Build history of the part. All positions in model axes, mm. Round coordinates to 2 decimals unless told otherwise and drop trailing zeros. Loops run counter-clockwise (first coordinate to the right, second up) from the corner with the lowest first, then second, coordinate; pieces in that order, holes last. Notation, with made-up numbers: (78, 64) - (114, 64) arc R11 ccw to (114, 80) - close; hole circle Ø7 at (63.25, -1). An arc over 180 degrees is marked (long way). Put each result on its own line as item: value. Start each with the question number.
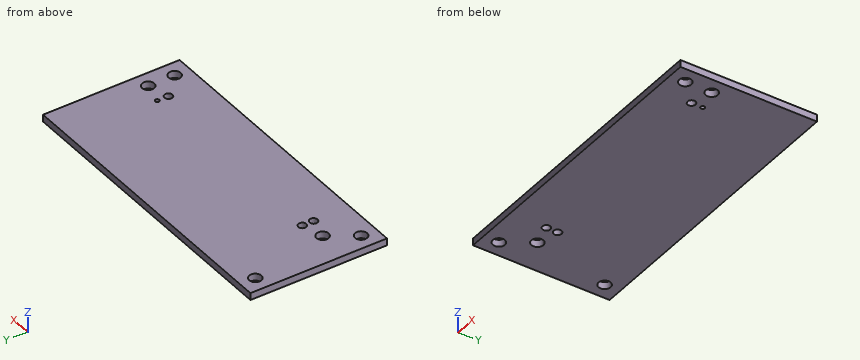
Autodesk Inventor part; units mm, degrees
ref_plane "YZ Plane" through (0, 0, 0) normal (1, 0, 0) x (0, 1, 0)
ref_plane "XZ Plane" through (0, 0, 0) normal (0, 1, 0) x (-1, 0, 0)
ref_plane "XY Plane" through (0, 0, 0) normal (0, 0, 1) x (1, 0, 0)
sketch "Sketch1" plane through (0, 0, 0) normal (0, 0, 1) x (1, 0, 0)
  line L0 (0, -53) -> (79, -53)
  line L1 (82, -50) -> (82, 0)
  circle A0 centre (78.5, -49.5) radius 1.375
  circle A1 centre (20.5, -49.5) radius 1.375
  line L2 (35.3891, -15.1062) -> (35.3891, -19.5)
  line L3 (35.3891, -19.5) -> (38.2391, -19.5)
  line L4 (38.2391, -19.5) -> (38.2391, -16.9)
  line L5 (38.2391, -16.9) -> (36.6891, -16.9)
  line L6 (36.6891, -16.9) -> (36.6891, -0.1)
  line L7 (36.6891, -0.1) -> (38.2391, -0.1)
  line L8 (38.2391, -0.1) -> (38.2391, 2.5)
  line L9 (38.2391, 2.5) -> (35.3891, 2.5)
  line L10 (35.3891, 2.5) -> (35.3891, -1.8938)
  line L11 (35.3891, -1.8938) -> (34.3391, -2.5)
  line L12 (34.3391, -2.5) -> (34.3391, -14.5)
  line L13 (34.3391, -14.5) -> (35.3891, -15.1062)
  line L14 (12.09, -50.25) -> (12.09, -37.75)
  circle A2 centre (25.37, -48.23) radius 0.9016
  circle A3 centre (25.37, -50.77) radius 0.9016
  circle A4 centre (73.63, -50.77) radius 0.9016
  circle A5 centre (73.63, -48.23) radius 0.474
  line L15 (13, -59) -> (82, -59)
  line L16 (82, -59) -> (82, -28)
  line L17 (82, -28) -> (13, -28)
  line L18 (13, -28) -> (13, -59)
  circle A6 centre (16.5, -55.5) radius 1.375
  circle A7 centre (16.5, -31.5) radius 1.375
  circle A8 centre (78.5, -55.5) radius 1.375
  point P0 (0, 0)
  dimension "d0" = 69
  dimension "d1" = 6
  dimension "d2" = 25
  dimension "d3" = 2.75
  dimension "d4" = 3.5
  dimension "d5" = 3.5
  dimension "d6" = 2.75
  dimension "d7" = 3.5
  dimension "d8" = 3.5
  dimension "d9" = 2.75
  dimension "d10" = 3.5
  dimension "d11" = 3.5
extrude "Extrusion1" add sketch "Sketch1" along normal blind 1.6 contours L16 L15 L18 L17 L1
properties part number "ShieldBare"
1) Slice it at C-C, the plane y = -55.5. Write the cut outline in (x, z) (3 decimals), and give its area (3 significant figures).
2) Drop a flat-ended pin along its axis: pin 1 Ø1.6 at (x, y) = (20.5, -49.5) entering from +Z. Give the stop position or say it passes through.
3) Slice it at A-A, the plane x = 16.5. Write the cut outline in (y, z) (3 decimals), and give its area (3 significant figures).
4) Drill centre lines: line 1 (Y direction, x = 16.5, z = 0.5) (3 decimals); line 2 (Y direction, x = 25.5, z = 0.6); line 3 (X direction, y = -49, z = 1.3). Where is each one in solid material? Low to high. Write a range as [from, to].
5) Slice it at B-B, the plane z = 0.45. State how many separate pieces and enclosed holes the cut face has, and give its area (3 significant figures).
Taken from the geometry:
1. outline: (13, 0) - (15.125, 0) - (15.125, 1.6) - (13, 1.6) - close; (17.875, 0) - (77.125, 0) - (77.125, 1.6) - (17.875, 1.6) - close; (79.875, 0) - (82, 0) - (82, 1.6) - (79.875, 1.6) - close
1. area: 102 mm2
2. pin 1: passes through
3. outline: (-59, 0) - (-56.875, 0) - (-56.875, 1.6) - (-59, 1.6) - close; (-54.125, 0) - (-32.875, 0) - (-32.875, 1.6) - (-54.125, 1.6) - close; (-30.125, 0) - (-28, 0) - (-28, 1.6) - (-30.125, 1.6) - close
3. area: 40.8 mm2
4. line 1: y = [-59, -56.875], [-54.125, -32.875], [-30.125, -28]
4. line 2: y = [-59, -51.66], [-49.88, -49.12], [-47.34, -28]
4. line 3: x = [13, 19.22], [21.78, 24.9], [25.84, 77.22], [79.78, 82]
5. separate pieces: 1
5. enclosed holes: 9
5. area: 2,100 mm2
